Model file for the job. Use its own axes, mm. Coordinates: 2 decimals unless noted, no trailing zeros. Loops run counter-clockwise (first coordinate to the right, second up) from the corner with the lowest first, then second, coordinate; pieces in that order, holes last.
from build123d import *

# Parameters (mm, degrees)
CROQUIS1_R              = 1.5
CROQUIS1_R_2            = 4
CROQUIS1_R_3            = 4.5
SALIENTE_EXTRUIR1_DEPTH = 6


with BuildPart() as part:
    # Croquis1 → Saliente-Extruir1 (new body)
    with BuildSketch(Plane.XY):
        with BuildLine():
            ThreePointArc((-166.230647244, 74.874670253), (-162.695113338, 76.339136347), (-161.230647244, 79.874670253))
            Line((-161.230647244, 79.874670253), (-161.230647244, 86.870701075))
            ThreePointArc((-161.230647244, 86.870701075), (-162.039949935, 89.59798105), (-164.20586967, 91.442383017))
            Line((-164.20586967, 91.442383017), (-189.641602091, 102.707755643))
            ThreePointArc((-189.641602091, 102.707755643), (-190.150317176, 102.968821046), (-190.625899632, 103.286260034))
            Line((-190.625899632, 103.286260034), (-243.282498112, 142.965853083))
            ThreePointArc((-243.282498112, 142.965853083), (-245.323514753, 145.031918552), (-246.684791002, 147.597323475))
            ThreePointArc((-246.684791002, 147.597323475), (-249.33333249, 155.226277836), (-253.46024382, 162.167770437))
            ThreePointArc((-253.46024382, 162.167770437), (-255.706791789, 164.36963499), (-258.526200935, 165.764668091))
            ThreePointArc((-258.526200935, 165.764668091), (-267.807267276, 167.484933762), (-277.233031605, 166.98246665))
            ThreePointArc((-277.233031605, 166.98246665), (-280.839635864, 165.006508056), (-281.744934312, 160.994969527))
            ThreePointArc((-281.744934312, 160.994969527), (-279.629843944, 151.795844616), (-275.418009863, 143.348480526))
            ThreePointArc((-275.418009863, 143.348480526), (-273.299883496, 141.022813744), (-270.564082899, 139.470209357))
            ThreePointArc((-270.564082899, 139.470209357), (-262.753961023, 137.416502238), (-254.690502443, 136.973385563))
            ThreePointArc((-254.690502443, 136.973385563), (-251.84925837, 136.371964278), (-249.300648344, 134.979497983))
            Line((-249.300648344, 134.979497983), (-196.590704681, 95.259706455))
            ThreePointArc((-196.590704681, 95.259706455), (-196.340024178, 95.057833866), (-196.102851224, 94.840251132))
            Line((-196.102851224, 94.840251132), (-177.15641917, 76.300948025))
            ThreePointArc((-177.15641917, 76.300948025), (-175.547795242, 75.244950437), (-173.659490598, 74.874670253))
            Line((-173.659490598, 74.874670253), (-166.230647244, 74.874670253))
        make_face()
        with Locations((-169.217002345, 80.892820484)):
            Circle(CROQUIS1_R, mode=Mode.SUBTRACT)
        with Locations((-176.480647244, 90.124670253)):
            Circle(CROQUIS1_R_2, mode=Mode.SUBTRACT)
        with Locations((-186.790930649, 94.135725334)):
            Circle(CROQUIS1_R, mode=Mode.SUBTRACT)
        with Locations((-205.155600297, 107.974496526)):
            Circle(CROQUIS1_R, mode=Mode.SUBTRACT)
        with BuildLine():
            Line((-261.989778965, 145.534030037), (-261.600094282, 142.761279445))
            ThreePointArc((-261.600094282, 142.761279445), (-262.876736734, 141.06711769), (-264.570898489, 142.343760142))
            Line((-264.570898489, 142.343760142), (-264.960583171, 145.116510734))
            ThreePointArc((-264.960583171, 145.116510734), (-263.68394072, 146.810672489), (-261.989778965, 145.534030037))
        make_face(mode=Mode.SUBTRACT)
        with BuildLine():
            Line((-271.680758131, 150.180525793), (-274.453508724, 149.79084111))
            ThreePointArc((-274.453508724, 149.79084111), (-276.147670478, 151.067483562), (-274.871028026, 152.761645316))
            Line((-274.871028026, 152.761645316), (-272.098277434, 153.151329999))
            ThreePointArc((-272.098277434, 153.151329999), (-270.404115679, 151.874687547), (-271.680758131, 150.180525793))
        make_face(mode=Mode.SUBTRACT)
        with Locations((-264.51202067, 152.702767498)):
            Circle(CROQUIS1_R_3, mode=Mode.SUBTRACT)
        with BuildLine():
            Line((-257.34328321, 155.225009203), (-254.570532617, 155.614693886))
            ThreePointArc((-254.570532617, 155.614693886), (-252.876370863, 154.338051434), (-254.153013314, 152.64388968))
            Line((-254.153013314, 152.64388968), (-256.925763907, 152.254204997))
            ThreePointArc((-256.925763907, 152.254204997), (-258.619925661, 153.530847449), (-257.34328321, 155.225009203))
        make_face(mode=Mode.SUBTRACT)
        with Locations((-274.894282301, 160.526362799)):
            Circle(CROQUIS1_R_2, mode=Mode.SUBTRACT)
        with BuildLine():
            Line((-267.034262376, 159.871504959), (-267.423947058, 162.644255551))
            ThreePointArc((-267.423947058, 162.644255551), (-266.147304607, 164.338417306), (-264.453142852, 163.061774854))
            Line((-264.453142852, 163.061774854), (-264.063458169, 160.289024262))
            ThreePointArc((-264.063458169, 160.289024262), (-265.340100621, 158.594862507), (-267.034262376, 159.871504959))
        make_face(mode=Mode.SUBTRACT)
    extrude(amount=SALIENTE_EXTRUIR1_DEPTH)


solid = part.part
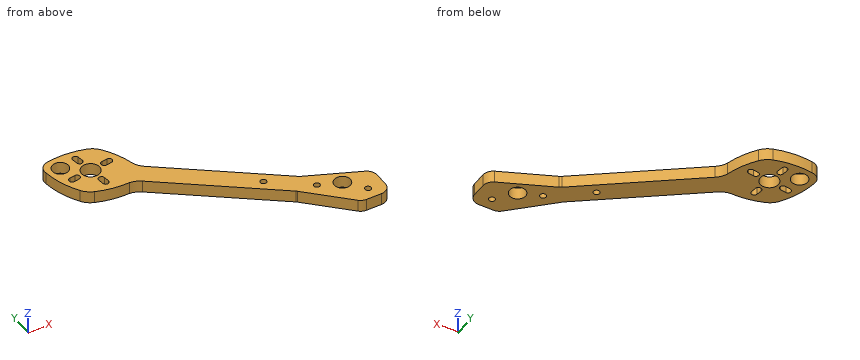
Q1. Slice it at C-C (y = 120.5). List the corners of the cut face in (x, z).
Answers:
outline: (-230.09, 0) - (-213.47, 0) - (-213.47, 6) - (-230.09, 6) - close
Q2. Flat gauge pins, fed straight in: P1, Ø8, axis at x = -206, y = 115.5, coming from the +Z side; P2, Ø1.5, axis at y = 93.5, z = 4.5, coming from the +X side. Where does each tip first touch, or does it go through?
Answers:
P1: stops at z = 6
P2: stops at x = -167.16
Q3. Slice it at D-D (x = -200.5). List the corners of the cut face in (y, z), and give its area (3 significant figures).
Answers:
outline: (98.21, 0) - (110.73, 0) - (110.73, 6) - (98.21, 6) - close
area: 75.1 mm2
Q4. Slice it at A-A (x = -175.5). List the corners of the cut face in (y, z).
Answers:
outline: (75.23, 0) - (86.25, 0) - (86.25, 6) - (75.23, 6) - close; (94, 0) - (96.44, 0) - (96.44, 6) - (94, 6) - close
Q5. Drill centre lines: line 1 (X direction, y = 154, z = 3.85); line 2 (X direction, y = 163, z = 2.9); line 3 (Y direction, x = -174, z = 1.45). Where is each one in solid material? Low to high.
Answers:
line 1: x = -280.35 to -268.82, -260.2 to -258.61, -252.87 to -248.79
line 2: x = -281.74 to -278.04, -271.75 to -267.43, -264.44 to -254.15
line 3: y = 74.89 to 86.99, 93.26 to 95.78
Q6. Slice it at B-B (z = 1.2). Count the separate pieces of the cut face and the enclosed holes in it, and give its area (3 significant figures).
Answers:
separate pieces: 1
enclosed holes: 10
area: 1,850 mm2
